Input: part model. Units: mm. Frame: model coordinates. A direction names the side the tool comes from. Round coordinates to 2 decimals unless told otherwise and drop trailing zeros. Loops run counter-clockwise (first coordinate to the right, second up) from the corner with the lowest first, then second, coordinate; pieces in that order, holes last.
1) Section B-B, the plane x = 22.75. Return loops of the section in (y, z), and give its area (3 significant figures).
2) Section C-C, the plane z = 9. Return loops of the section in (x, y), and give its area (3 significant figures).
3) Section D-D, the plane x = 39.5. Return loops of the section in (y, z), and give its area (3 significant figures).
4) First-contact query: pin 1 (0.6 mm diameter, centred on y = 52, z = 3, fed in from -X); pin 2 (0.6 mm diameter, centred on x = 37.5, y = 52.5, fed in from -Z); pin 3 (0.6 mm diameter, centred on x = 50, y = 39.5, fed in from -Z); pin 4 (2 mm diameter, centred on x = 30, z = 3.5, fed in from -Y). Flat tips, straight axial feed; report the tip coordinate or a pass-through.
5) Section A-A, the plane y = 50. Return loops of the section in (x, z), and give its area (3 significant figures).
6) Ray query, line 1 along Y through (x, z) = (22.75, 11.85); line 2 along Y through (x, z) = (6.5, 9.75); line 3 along Y through (x, z) = (22.75, 5). Return the intervals inside material, ascending.
7) Access query for faces 1 (the face through (50, 27, 4.7)), 2 (the face through (50, 45.5, 5)), 3 (the face through (30, 1, 5.15)). Directions: +Z, -Z, +X, -X, +Y, -Y. A direction counts if a zero-diameter tool reaches every point of the face in a straight line with its end or side. Return the directions, or none.
8) Draft query along Y for faces 4 (the face through (26.15, 48, 8)), 5 (the face through (2, 26, 6)), 6 (the face through (50, 49, 2)). Return one class per face: pulls with the +Y half, pulls with the -Y half, needs draft (parallel to the pull), parting line crosses it, or undercut.
from build123d import *

# Parameters (mm, degrees)
EXTRUDE024_DEPTH = 8
EXTRUDE023_DEPTH = 10
SKETCH017_W      = 8.15
SKETCH017_H      = 2.65
EXTRUDE013_DEPTH = 2
SKETCH016_R      = 1.2
EXTRUDE012_DEPTH = 10
SKETCH010_W      = 14.7
SKETCH010_H      = 2.65
SKETCH010_W_2    = 23.15
SKETCH010_H_2    = 3.15
EXTRUDE006_DEPTH = 53
SKETCH011_W      = 15.2
SKETCH011_H      = 2.7
EXTRUDE007_DEPTH = 51.25
SKETCH009_W      = 51.25
SKETCH009_H      = 53
SKETCH009_W_2    = 47.25
SKETCH009_H_2    = 49
EXTRUDE004_DEPTH = 10
SKETCH008_W      = 51.25
SKETCH008_H      = 53
EXTRUDE003_DEPTH = 2
SKETCH028_W      = 5
SKETCH028_H      = 5
EXTRUDE025_DEPTH = 5


with BuildPart() as cuts003:
    # Sketch027 → Extrude024 (new body)
    with BuildSketch(Plane.XZ):
        with BuildLine():
            Line((49.15, 2), (53.120454, 2))
            ThreePointArc((53.120454, 2), (52.24615, 3.831644), (51.25, 5.59998))
            Line((51.25, 8), (51.25, 5.59998))
            Line((51.25, 8), (49.15, 8))
            Line((49.15, 8), (49.15, 2))
        make_face()
    extrude(amount=-EXTRUDE024_DEPTH)


with BuildPart() as cuts003_1:
    # Extrude024 placement: moved
    add(cuts003.part.moved(Location((0, 37.5, 0))))


with BuildPart() as topcut001:
    # Sketch026 → Extrude023 (new body)
    with BuildSketch(Plane.XZ):
        with BuildLine():
            Line((49.15, 2), (53.120454, 2))
            ThreePointArc((53.120454, 2), (52.24615, 3.831644), (51.25, 5.59998))
            Line((51.25, 8), (51.25, 5.59998))
            Line((51.25, 8), (49.15, 8))
            Line((49.15, 8), (49.15, 2))
        make_face()
    extrude(amount=-EXTRUDE023_DEPTH)


with BuildPart() as topcut001_1:
    # Extrude023 placement: moved
    add(topcut001.part.moved(Location((0, 7.5, 0))))

    # Fusion005: union cuts003
    add(cuts003_1.part)


with BuildPart() as extrude013:
    # Sketch017 → Extrude013 (new body)
    with BuildSketch(Plane.XZ):
        with Locations((37.575, 6.475)):
            Rectangle(SKETCH017_W, SKETCH017_H)
    extrude(amount=-EXTRUDE013_DEPTH)


with BuildPart() as topcut:
    # Sketch016 → Extrude012 (new body)
    with BuildSketch(Plane.XY):
        with Locations((22.75, 50)):
            Circle(SKETCH016_R)
        with Locations((22.75, 3.25)):
            Circle(SKETCH016_R)
    extrude(amount=-EXTRUDE012_DEPTH)


with BuildPart() as topcut_1:
    # Extrude012 placement: moved
    add(topcut.part.moved(Location((0, 0, 12.25))))


with BuildPart() as topcuts:
    # Sketch010 → Extrude006 (new body)
    with BuildSketch(Plane.XZ):
        with Locations((10.5, 3.325)):
            Rectangle(SKETCH010_W, SKETCH010_H)
        with Locations((37.575, 3.575)):
            Rectangle(SKETCH010_W_2, SKETCH010_H_2)
    extrude(amount=-EXTRUDE006_DEPTH)


with BuildPart() as fusion001:
    # Sketch011 → Extrude007 (new body)
    with BuildSketch(Plane.YZ):
        with Locations((27.5, 3.35)):
            Rectangle(SKETCH011_W, SKETCH011_H)
    extrude(amount=EXTRUDE007_DEPTH)

    # Fusion001: union topCuts
    add(topcuts.part)


with BuildPart() as top:
    # Sketch009 → Extrude004 (new body)
    with BuildSketch(Plane.XY):
        with Locations((25.625, 26.5)):
            Rectangle(SKETCH009_W, SKETCH009_H)
        with Locations((25.625, 26.5)):
            Rectangle(SKETCH009_W_2, SKETCH009_H_2, mode=Mode.SUBTRACT)
    extrude(amount=EXTRUDE004_DEPTH)


with BuildPart() as top_1:
    # Extrude004 placement: moved
    add(top.part.moved(Location((0, 0, 2))))


with BuildPart() as top005:
    # Sketch008 → Extrude003 (new body)
    with BuildSketch(Plane.XY):
        with Locations((25.625, 26.5)):
            Rectangle(SKETCH008_W, SKETCH008_H)
    extrude(amount=EXTRUDE003_DEPTH)


with BuildPart() as top005_1:
    # Extrude003 placement: moved
    add(top005.part.moved(Location((0, 0, 10.25))))

    # Fusion: union top
    add(top_1.part)

    # Cut001: cut Fusion001
    add(fusion001.part, mode=Mode.SUBTRACT)

    # Cut003: cut topCut
    add(topcut_1.part, mode=Mode.SUBTRACT)

    # Cut005: cut Extrude013
    add(extrude013.part, mode=Mode.SUBTRACT)


with BuildPart() as top008:
    # Sketch028 → Extrude025 (new body)
    with BuildSketch(Plane.XY.offset(10.25)):
        with Locations((28.65, 48.5)):
            Rectangle(SKETCH028_W, SKETCH028_H)
        with Locations((46.75, 48.5)):
            Rectangle(SKETCH028_W, SKETCH028_H)
    extrude(amount=-EXTRUDE025_DEPTH)

    # Fusion006: union top005
    add(top005_1.part)

    # Cut: cut topCut001
    add(topcut001_1.part, mode=Mode.SUBTRACT)


solid = top008.part
Final values:
1. outline: (0, 2) - (2, 2) - (2, 10.25) - (2.05, 10.25) - (2.05, 12.25) - (0, 12.25) - close; (4.45, 10.25) - (48.8, 10.25) - (48.8, 12.25) - (4.45, 12.25) - close; (51, 2) - (53, 2) - (53, 12.25) - (51.2, 12.25) - (51.2, 2.25) - (51, 2.25) - close
1. area: 128 mm2
2. outline: (0, 0) - (51.25, 0) - (51.25, 53) - (0, 53) - close; hole (2, 2) - (49.25, 2) - (49.25, 46) - (44.25, 46) - (44.25, 51) - (31.15, 51) - (31.15, 46) - (26.15, 46) - (26.15, 51) - (23.41, 51) arc R1.2 ccw to (22.09, 51) - (2, 51) - close
2. area: 451 mm2
3. outline: (0, 7.8) - (2, 7.8) - (2, 10.25) - (51, 10.25) - (51, 5.15) - (53, 5.15) - (53, 12.25) - (0, 12.25) - close
3. area: 121 mm2
4. pin 1: stops at x = 0
4. pin 2: stops at z = 5.15
4. pin 3: stops at z = 8
4. pin 4: passes through
5. outline: (0, 2) - (2, 2) - (2, 10.25) - (21.55, 10.25) - (21.55, 12.25) - (0, 12.25) - close; (23.95, 10.25) - (26.15, 10.25) - (26.15, 5.25) - (31.15, 5.25) - (31.15, 10.25) - (44.25, 10.25) - (44.25, 5.25) - (49.25, 5.25) - (49.25, 2) - (51.25, 2) - (51.25, 12.25) - (23.95, 12.25) - close
5. area: 181 mm2
6. line 1: y = 0 to 2.05, 4.45 to 48.8, 51.2 to 53
6. line 2: y = 0 to 2, 51 to 53
6. line 3: y = 0 to 2, 51.2 to 53
7. face 1: -Z, +X, -X
7. face 2: -Z, +X
7. face 3: -Z, +Y, -Y
8. face 4: undercut
8. face 5: undercut
8. face 6: needs draft
